Check sheet for the modelled part. Datum: model origin and axes. Units: mm. Face numbers are marked on the shaded views. A direction names the side the tool comes from. Give positions to 0.01 mm unless a question says otherwise; leave off trailing zeros. Loops run counter-clockwise (first coordinate to the right, second up) from the corner with the lowest first, then second, coordinate; pieces in that order, holes last. Notation, with made-up numbers: M 46,24 L 71,24 A12 cw 71,44 Z; hole C 15.5,-10 d11. An arc over 180 degrees is marked long. Use one line per item in the form item = value.
from build123d import *

# Parameters (mm, degrees)
SKETCH1_R                 = 3
BOSS_EXTRUDE1_DEPTH       = 10
M3X0_5_TAPPED_HOLE1_D     = 2.5
M3X0_5_TAPPED_HOLE1_DEPTH = 5
M3X0_5_TAPPED_HOLE1_TIP   = 0.751075774


with BuildPart() as part:
    # Sketch1 → Boss-Extrude1 (new body)
    with BuildSketch(Plane(origin=(0, 0, 0), x_dir=(1, 0, 0), z_dir=(0, 1, 0))):
        Polygon((23.48448278, 27.298019474), (33.48448278, 27.298019474), (33.48448278, 37.298019474), (43.48448278, 37.298019474), (43.48448278, 27.298019474), (70.48448278, 27.298019474), (70.48448278, -12.701980526), (-40.51551722, -12.701980526), (-40.51551722, 27.298019474), (13.48448278, 27.298019474), (13.48448278, 37.298019474), (23.48448278, 37.298019474), align=None)
        with Locations(Location((-34.51551722, -6.701980526, 0), (0, 0, 270))):
            Circle(SKETCH1_R, mode=Mode.SUBTRACT)
        with Locations(Location((-9.51551722, -6.701980526, 0), (0, 0, 270))):
            Circle(SKETCH1_R, mode=Mode.SUBTRACT)
        with Locations(Location((15.48448278, -6.701980526, 0), (0, 0, 270))):
            Circle(SKETCH1_R, mode=Mode.SUBTRACT)
    extrude(amount=BOSS_EXTRUDE1_DEPTH)

    # M3x0.5 Tapped Hole1
    with Locations(Plane(origin=(0, 0, -27.298019474), x_dir=(-1, 0, 0), z_dir=(0, 0, -1))):
        with Locations((-28.48448278, 5)):
            Hole(M3X0_5_TAPPED_HOLE1_D / 2, depth=M3X0_5_TAPPED_HOLE1_DEPTH)
            with Locations((0, 0, -(M3X0_5_TAPPED_HOLE1_DEPTH + M3X0_5_TAPPED_HOLE1_TIP / 2))):  # 118° drill point
                Cone(0, M3X0_5_TAPPED_HOLE1_D / 2, M3X0_5_TAPPED_HOLE1_TIP, mode=Mode.SUBTRACT)


solid = part.part
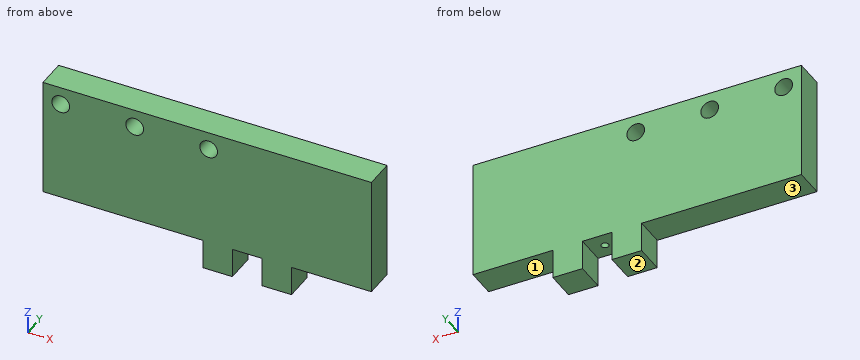
1) Scan lines: line 1 (X direction, y = 1.75, z = 7); line 2 (X direction, y = 0.5, z = 6); line 3 (X direction, y = 0.5, z = -31). Record each from-to range of solid material in increasing order.
Evaluation:
line_1 = -40.52 to -37.5, -31.53 to -12.5, -6.53 to 12.5, 18.47 to 70.48
line_2 = -40.52 to -37.43, -31.6 to -12.43, -6.6 to 12.57, 18.4 to 70.48
line_3 = 13.48 to 23.48, 33.48 to 43.48
2) Section check A-A (x = 62). Record the cut outline in (y, z).
Evaluation:
outline = M 0,-27.3 L 10,-27.3 L 10,12.7 L 0,12.7 Z
3) Depth check by flat-ended pin: pin 1 Ø5 at (x, y) = (57.5, 5) entering from -Z. Enter the tip coordinate at first touch or a pass-through.
Evaluation:
pin_1 = -27.3
4) Set-up check for the marked faces 1, 2 and 3: record each of +Z, -Z, +X, -X, +Y, -Y from which the full face is reachable in a straight line by a thin tool's end or side.
Evaluation:
face_1 = -Z, +X, +Y, -Y
face_2 = -Z, +X, -X, +Y, -Y
face_3 = -Z, -X, +Y, -Y
